Check sheet for the drawn part. Datum: minimum x, y, z corner. Units: mm. A direction names the side the tool comes from. Coordinates: 2 decimals unless noted, no trailing zeros. Order: outer loops, then holes, each group sorted by start corner. A loop starts at its lowest first (then second) coordinate and runs counter-clockwise, first axis right, second up. Notation, with made-up numbers: M 3,-20.5 L 35,-20.5 A29 cw 35,11.5 Z; hole C 54,51.5 d4. An arc over 180 degrees is marked long. Answer in a Markdown table with one row per item. Add a question column.
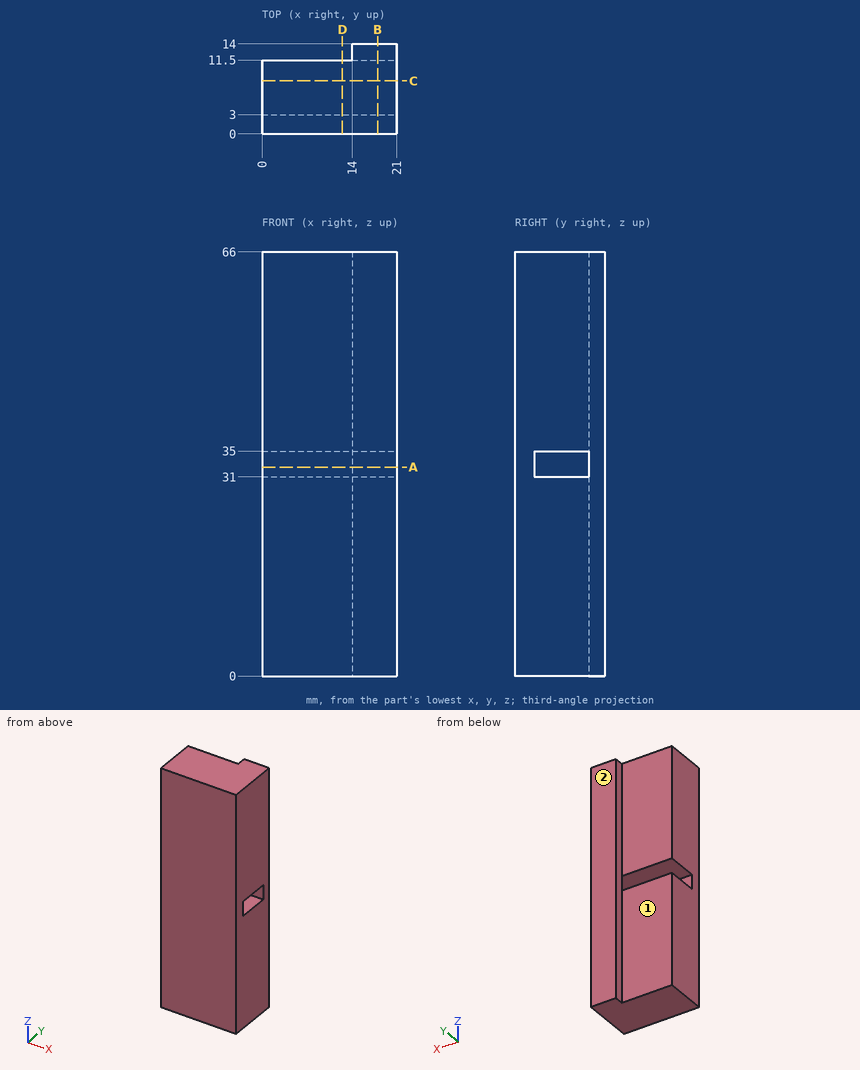
1. Go/stop test with a flat-tipped pin: pin 1 Ø11 at (x, z) = (4, 10) entering from +Y. Record where the tip stops, or that it passes through.
2. Scan lines: line 1 (Z direction, x = 19, y = 11); line 2 (Y direction, x = 5.75, z = 13); line 3 (X direction, y = 13, z = 20.5). Record each from-to range of solid material in increasing order.
3. Section check A-A on z = 32.5. Enter the section's corners in (x, y), then the cut area to 3 significant figures.
4. Section check B-B on x = 18. Enter the section's corners in (y, z).
5. Section check D-D on x = 12.5. Enter the section's corners in (y, z), then the cut area to 3 significant figures.
6. Set-up check for the marked faces 1 and 2: record each of +Z, -Z, +X, -X, +Y, -Y from which the full face is reachable in a straight line by a thin tool's end or side.
7. Section check C-C on y = 8.25. Enter the section's corners in (x, z).
Result sheet:
| question | item | result |
|---|---|---|
| 1 | pin 1 | y = 11.5 |
| 2 | line 1 | 0 to 31, 35 to 66 |
| 2 | line 2 | 0 to 11.5 |
| 2 | line 3 | 14 to 21 |
| 3 | outline | M 0,0 L 21,0 L 21,3 L 0,3 Z; M 14,11.5 L 21,11.5 L 21,14 L 14,14 Z |
| 3 | area | 80.5 mm^2 |
| 4 | outline | M 0,0 L 14,0 L 14,66 L 0,66 Z; hole M 3,31 L 11.5,31 L 11.5,35 L 3,35 Z |
| 5 | outline | M 0,0 L 11.5,0 L 11.5,31 L 3,31 L 3,35 L 11.5,35 L 11.5,66 L 0,66 Z |
| 5 | area | 725 mm^2 |
| 6 | face 1 | +Z, -Z, -X, +Y |
| 6 | face 2 | +Z, -Z, +X, -X, +Y |
| 7 | outline | M 0,0 L 21,0 L 21,31 L 0,31 Z; M 0,35 L 21,35 L 21,66 L 0,66 Z |
